Build history of the part. All positions in model axes, mm. Face numbers are marked on the shaded views. A direction names the side the tool comes from. Coordinates: 2 decimals unless noted, no trailing zeros. Loops run counter-clockwise (first coordinate to the right, second up) from the corner with the lowest first, then second, coordinate; pieces in that order, holes last. Notation, with made-up numbers: (67, 31.5) - (117, 31.5) arc R16 cw to (117, 61.5) - close; hole circle Ø1 at (56.25, -35.75). An arc over 180 degrees is marked (long way). One line per item, written item: value.
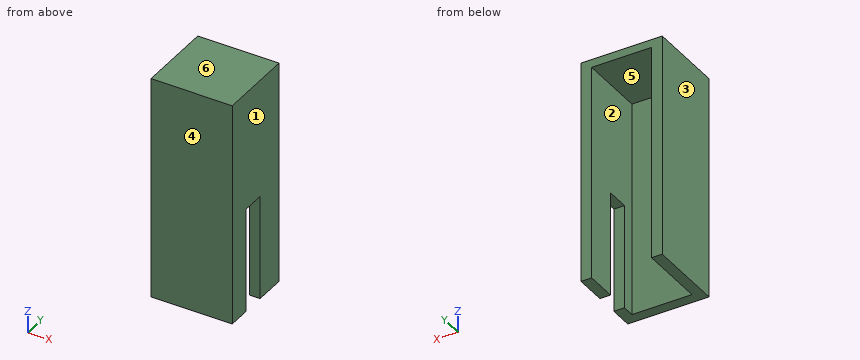
```python
from build123d import *

# Parameters (mm, degrees)
BOSS_EXTRUDE1_DEPTH = 42
SKETCH2_W           = 30.5
SKETCH2_H           = 29
BOSS_EXTRUDE2_DEPTH = 3
SKETCH3_W           = 40
SKETCH3_H           = 8.69
CUT_EXTRUDE1_DEPTH  = 30


with BuildPart() as part:
    # Sketch1 → Boss-Extrude1 (new body, symmetric)
    with BuildSketch(Plane.XY):
        Polygon((-9.848648649, 0), (-9.848648649, -25), (12.651351351, -25), (12.651351351, 0), (16.651351351, 0), (16.651351351, -29), (-13.848648649, -29), (-13.848648649, 0), align=None)
    extrude(amount=BOSS_EXTRUDE1_DEPTH, both=True)

    # Sketch2 → Boss-Extrude2 (add)
    with BuildSketch(Plane.XY.offset(42)):
        with Locations((1.401351351, -14.5)):
            Rectangle(SKETCH2_W, SKETCH2_H)
    extrude(amount=-BOSS_EXTRUDE2_DEPTH)

    # Sketch3 → Cut-Extrude1 (cut)
    with BuildSketch(Plane(origin=(0, 0, 0), x_dir=(0, 0, -1), z_dir=(1, 0, 0))):
        with Locations((22.65905185, -16.052995557)):
            Rectangle(SKETCH3_W, SKETCH3_H)
    extrude(amount=CUT_EXTRUDE1_DEPTH, mode=Mode.SUBTRACT)


solid = part.part
```
Item 1: Cut at B-B, the plane y = -17. Write the cut outline in (x, z), then the cut area to 3 significant figures.
Check result:
outline: (-13.85, -42) - (-9.85, -42) - (-9.85, 39) - (12.65, 39) - (12.65, -2.66) - (16.65, -2.66) - (16.65, 42) - (-13.85, 42) - close
area: 582 mm^2
Item 2: Probe probe 1 along Y at (x, z) = (14, -24); probe 2 along X at (y, z) = (-24, -34.5); probe 3 along Y at (x, z) = (-6, -33). List the from-to ranges inside material, lowest first. Write a range as from..to.
Check result:
probe 1: y = -29..-20.4, -11.71..0
probe 2: x = -13.85..-9.85, 12.65..16.65
probe 3: y = -29..-25
Item 3: Cut at D-D, the plane x = 5.5. Write the cut outline in (y, z).
Check result:
outline: (-29, -42) - (-25, -42) - (-25, 39) - (0, 39) - (0, 42) - (-29, 42) - close
Item 4: Cut at A-A, the plane z = -16. Write the cut outline in (x, y).
Check result:
outline: (-13.85, -29) - (16.65, -29) - (16.65, -20.4) - (12.65, -20.4) - (12.65, -25) - (-9.85, -25) - (-9.85, 0) - (-13.85, 0) - close; (12.65, -11.71) - (16.65, -11.71) - (16.65, 0) - (12.65, 0) - close
Item 5: Drop flat-ended pins along their axis: P1, Ø12, axis at x = 13.5, z = 25.5, coming from the +Y side; P2, Ø11, axis at x = 4.5, z = -7.5, coming from the +Y side; P3, Ø7, axis at x = 3.5, y = -7.5, coming from the -Z side; P4, Ø3, axis at x = 15.5, y = -17, coming from the -Z side. Give the stop position or say it passes through.
Check result:
P1: stops at y = 0
P2: stops at y = -25
P3: stops at z = 39
P4: stops at z = -2.66
Item 6: Pull direction X, two halves, no side cores. Call the marked faces 1, 2, 3 and 4: released by +X, released by -X, zero draft, split by the parting line, or undercut.
Check result:
face 1: released by +X
face 2: undercut
face 3: released by -X
face 4: zero draft
Item 7: Cut at C-C, the plane z = 36. Write the cut outline in (x, y).
Check result:
outline: (-13.85, -29) - (16.65, -29) - (16.65, 0) - (12.65, 0) - (12.65, -25) - (-9.85, -25) - (-9.85, 0) - (-13.85, 0) - close
Item 8: Tool access for the marked faces 5 and 6: list every direction of +Z, -Z, +X, -X, +Y, -Y with a clear straight run to the whole face (end or side of a thin tool).
Check result:
face 5: -Z, +Y
face 6: +Z, +X, -X, +Y, -Y
